Can you work these out from the drawing? Everything is in mm from the part's minimum corner. A direction names the side the tool comes from. Coordinates: 2 decimals unless noted, no trailing zeros. Write each loop counter-clockwise with the first axis right and the second up, starting at its lowest first coordinate (ties: lowest second). Pieces come first, ordered by that corner, then holes. Notation, with made-up numbers: M 25,88 L 74,88 A12 ccw 74,98 Z; hole C -18,14.25 d9. An arc over 180 degrees is marked long. Write item = value, one per line.
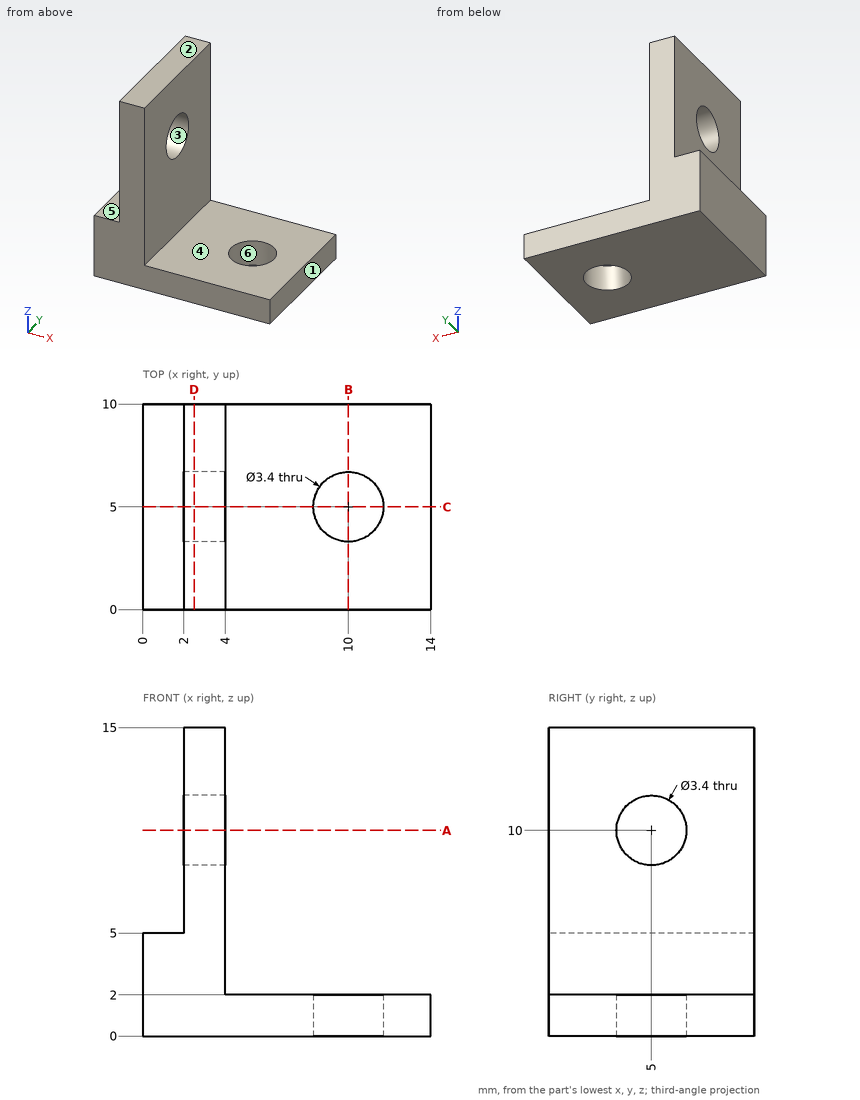
Item 1: If we mould it in two halves opening along Z, with no side actions, what happens to the marked faces 1, 2 and 3? For each: pulls with the +Z half, pulls with the -Z half, needs draft (parallel to the pull), parting line crosses it, or undercut.
Numbers:
face_1 = needs draft
face_2 = pulls with the +Z half
face_3 = undercut
Item 2: I'm going to push flat-ended pins straight in: P1, Ø3, axis at x = 6.5, z = 8, coming from the -Y side; P2, Ø4.5, axis at y = 5, z = 10, coming from the -X side; P3, Ø0.6, axis at x = 1.5, y = 6, coming from the +Z side; P4, Ø5, axis at x = 7, y = 5.5, coming from the +Z side. Where does each tip first touch, or does it pass through?
Numbers:
P1 = through
P2 = 2
P3 = 5
P4 = 2
Item 3: Imagine slicing it at A-A (z = 10). Write out the boundary of the cut face in (x, y), and give its area (3 significant figures).
Numbers:
outline = M 2,0 L 4,0 L 4,3.3 L 2,3.3 Z; M 2,6.7 L 4,6.7 L 4,10 L 2,10 Z
area = 13.2 mm²
Item 4: For the marked faces 4, 5 and 6, which set-ups out of +Z, -Z, +X, -X, +Y, -Y let a thin tool reach every point of the face, with its end or its side?
Numbers:
face_4 = +Z, +X, +Y, -Y
face_5 = +Z, -X, +Y, -Y
face_6 = +Z, -Z
Item 5: If I drill on line 1 along Z through (x, y) = (2.7, 5); line 2 along Y through (x, z) = (10, 0.85); line 3 along X through (y, z) = (5.25, 14.25), over which ranges is the centre line in solid material (lowest first)?
Numbers:
line_1 = 0 to 8.3, 11.7 to 15
line_2 = 0 to 3.3, 6.7 to 10
line_3 = 2 to 4
Item 6: Imagine slicing it at B-B (x = 10). Write out the boundary of the cut face in (y, z).
Numbers:
outline = M 0,0 L 3.3,0 L 3.3,2 L 0,2 Z; M 6.7,0 L 10,0 L 10,2 L 6.7,2 Z
Item 7: Imagine slicing it at D-D (x = 2.5). Write out the boundary of the cut face in (y, z), and give its area (3 significant figures).
Numbers:
outline = M 0,0 L 10,0 L 10,15 L 0,15 Z; hole C 5,10 d3.4
area = 141 mm²
Item 8: Imagine slicing it at C-C (y = 5). Write out the boundary of the cut face in (x, z).
Numbers:
outline = M 0,0 L 8.3,0 L 8.3,2 L 4,2 L 4,8.3 L 2,8.3 L 2,5 L 0,5 Z; M 2,11.7 L 4,11.7 L 4,15 L 2,15 Z; M 11.7,0 L 14,0 L 14,2 L 11.7,2 Z
